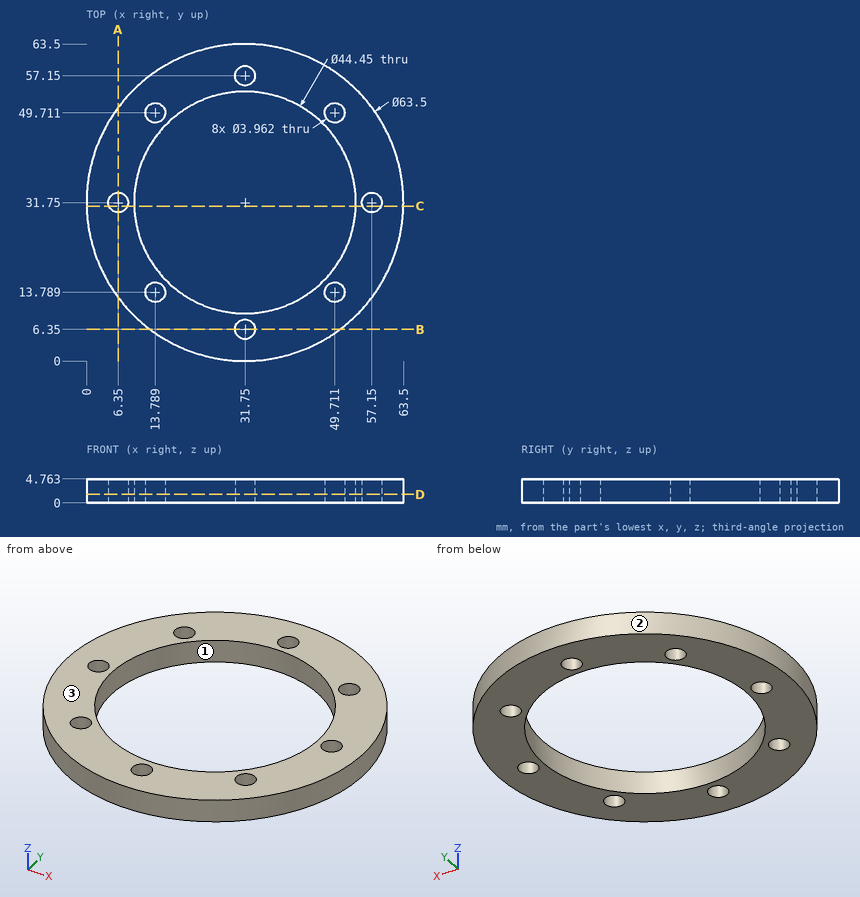
For this review, use the dimensioned drawing (mm, ordinates from the lowest corner) and the shaded views. Round coordinates to 2 decimals unless told otherwise and drop trailing zeros. Order: outer loops, then holes, each group sorted by start corner. A loop starts at its lowest first (then second) coordinate and runs counter-clockwise, first axis right, second up. Notation, with made-up numbers: (-29, -26) -> (20, -26) arc R14 cw to (20, -5) -> close; hole circle Ø2 at (51.25, 71). An arc over 180 degrees is marked (long way). Write item = value, one per line. Start each with the question number.
Item 1: Consider section D-D on z = 1.7. Count the separate pieces of the cut face and the enclosed holes in it, plus the area to 3 significant figures.
Item 2: Consider section A-A on x = 6.35. Write out the cut boundary in (y, z).
Item 3: Mouldability with a two-part tool opening along Y and no side actions: class the marked faces 1, 2 and 3 as released by +Y, released by -Y, zero draft, split by the parting line, or undercut.
Item 4: Consider section C-C on y = 31. Write out the cut boundary in (x, z).
Item 5: Clearance check with flat-ended pins moving along their axes: pin 1 Ø2 at (y, z) = (11.5, 1) entering from -X; pin 2 Ø1.5 at (y, z) = (40.5, 3.5) entering from +X (1 decimal). State where each tip first meets the part, or that it passes through.
Item 6: For line 1 along X through (y, z) = (49, 3.4) (1 decimal); line 2 along Y through (x, z) = (15.5, 0.9) (1 decimal); line 3 along X through (y, z) = (12, 3.2) (1 decimal), list the stretches that pass through material, from the lowest coordinate up.
Conclusion:
q1.separate_pieces = 1
q1.enclosed_holes = 9
q1.area = 1,520 mm2
q2.outline = (12.7, 0) -> (29.77, 0) -> (29.77, 4.76) -> (12.7, 4.76) -> close; (33.73, 0) -> (50.8, 0) -> (50.8, 4.76) -> (33.73, 4.76) -> close
q3.face_1 = undercut
q3.face_2 = split by the parting line
q3.face_3 = zero draft
q4.outline = (0.01, 0) -> (4.52, 0) -> (4.52, 4.76) -> (0.01, 4.76) -> close; (8.18, 0) -> (9.54, 0) -> (9.54, 4.76) -> (8.18, 4.76) -> close; (53.96, 0) -> (55.32, 0) -> (55.32, 4.76) -> (53.96, 4.76) -> close; (58.98, 0) -> (63.49, 0) -> (63.49, 4.76) -> (58.98, 4.76) -> close
q5.pin_1 = 6.5
q5.pin_2 = 62.5
q6.line_1 = 5.1 to 11.9, 15.6 to 17.7, 45.8 to 47.9, 51.6 to 58.4
q6.line_2 = 4.5 to 12.8, 14.8 to 16.6, 46.9 to 48.7, 50.7 to 59
q6.line_3 = 6.9 to 12.9, 14.6 to 21.6, 41.9 to 48.9, 50.6 to 56.6
